Can you work these out from the model? Positions are in its coordinate system, mm. A direction names the side the tool comes from. Give positions to 0.01 mm unless a question says otherwise; leave off trailing zeros. Order: outer loops, then holes, each group sorted by start corner. A loop starts at its lowest first (then second) coordinate and runs counter-clockwise, first axis right, second up. Notation, with made-up numbers: (42, 59) - (92, 59) arc R25 cw to (92, 77) - close; hole circle Ø9 at (-30.5, -19.75). An arc over 180 degrees is marked (long way). Answer as a JSON object with one key per item and string values.
Autodesk Inventor part; units mm, degrees
ref_plane "YZ Plane" through (0, 0, 0) normal (1, 0, 0) x (0, 1, 0)
ref_plane "XZ Plane" through (0, 0, 0) normal (0, 1, 0) x (-1, 0, 0)
ref_plane "XY Plane" through (0, 0, 0) normal (0, 0, 1) x (1, 0, 0)
sketch "Sketch1" plane through (0, 0, 0) normal (0, 0, 1) x (1, 0, 0)
  circle A0 centre (0, 0) radius 12.7
  circle A1 centre (0, 0) radius 15
  circle A2 centre (0, 0) radius 25.5
  circle A3 centre (0, 0) radius 27
  dimension "d1" = 25.4
  dimension "d2" = 30
  dimension "d3" = 51
  dimension "d4" = 54
extrude "Extrusion1" add sketch "Sketch1" along normal blind 15 contours A1
extrude "Extrusion2" add sketch "Sketch1" along normal blind 2 contours A2
extrude "Extrusion3" add sketch "Sketch1" along normal blind 2 and the other way blind 5 contours A3
equation "\"BendRadius\" = Thickness"
equation "\"BendReliefWidth\" = Thickness"
equation "\"BendReliefDepth\" = 0.5 * Thickness"
equation "\"CornerReliefSize\" = 4 * Thickness"
equation "\"MinimumRemnant\" = 2 * Thickness"
equation "\"TransitionRadius\" = BendRadius"
equation "\"JacobiRadiusSize\" = BendRadius"
equation "\"GapSize\" = Thickness"
Q1. I'm going to push flat-ended pins straight in: pin 1 Ø1.5 at (y, z) = (9.5, 9) entering from -X; pin 2 Ø10 at (x, z) = (14, 2.5) entering from +Y; pin 3 Ø2 at (y, z) = (2, 7) entering from -X. Where does each tip first touch, or does it pass through?
Recorded:
{"pin 1": "stops at x = -12.18", "pin 2": "stops at y = 25.45", "pin 3": "stops at x = -14.97"}
Q2. I need wall thicknesses on L1, parallel to Y at x = 0, z = 5; L2, parallel to Y at x = 0, z = -2.35; L3, parallel to Z at x = -16.5, y = -17. Which ranges of each line are inside material? Lowest first, please.
Recorded:
{"L1": "y = -15 to -12.7, 12.7 to 15", "L2": "y = -27 to -25.5, 25.5 to 27", "L3": "z = 0 to 2"}
Q3. We'd pull the mould along Y, two halves only. Please class faces 1 (the face through (-5.85, -26.36, -1.45)), 2 (the face through (-11, 7, 15)), 3 (the face through (5, 12, 0)): released by +Y, released by -Y, zero draft, split by the parting line, or undercut.
Recorded:
{"face 1": "split by the parting line", "face 2": "zero draft", "face 3": "undercut"}
Q4. If we section it at C-C, the plane z = 4: Please give me the cut outline in (x, y).
Recorded:
{"outline": "circle Ø30 at (0, 0); hole circle Ø25.4 at (0, 0)"}
Q5. If we section it at A-A, the plane y = 0: Please give me the cut outline in (x, z), then the cut area to 3 significant figures.
Recorded:
{"outline": "(-27, -5) - (-25.5, -5) - (-25.5, 0) - (-12.7, 0) - (-12.7, 15) - (-15, 15) - (-15, 2) - (-27, 2) - close; (12.7, 0) - (25.5, 0) - (25.5, -5) - (27, -5) - (27, 2) - (15, 2) - (15, 15) - (12.7, 15) - close", "area": "132 mm^2"}
Q6. If we section it at D-D, the plane x = -20: Please give me the cut outline in (y, z), then the cut area to 3 significant figures.
Recorded:
{"outline": "(-18.14, -5) - (-15.82, -5) - (-15.82, 0) - (15.82, 0) - (15.82, -5) - (18.14, -5) - (18.14, 2) - (-18.14, 2) - close", "area": "95.7 mm^2"}
Q7. Which directions (+Z, -Z, +X, -X, +Y, -Y) give clear straight access to the entire face, cutting with the end or side of a thin tool? Please do faces 4 (the face through (-5.5, -24.9, -2.5)), 5 (the face through (-14.985, -0.66, 8.409)), 6 (the face through (24, -10, -5)).
Recorded:
{"face 4": "-Z", "face 5": "+Z", "face 6": "-Z, +X, -X, +Y, -Y"}
